Geometry check sheet. Reference: the model listing, model coordinates, mm. A direction names the side the tool comes from. Round coordinates to 2 decimals unless told otherwise and drop trailing zeros. Order: outer loops, then holes, each group sorted by start corner. A loop starts at its lowest first (then second) coordinate and runs counter-clockwise, first axis right, second up.
```python
from build123d import *

# Parameters (mm, degrees)
SKETCH1_W           = 66
SKETCH1_H           = 49
BOSS_EXTRUDE1_DEPTH = 19
SHELL1_T            = -1.5
SKETCH2_W           = 6
SKETCH2_H           = 4.6
BOSS_EXTRUDE2_DEPTH = 17.5
FILLET1_R           = 1.5
SKETCH3_R           = 2.15
SKETCH3_R_2         = 1.45
BOSS_EXTRUDE3_DEPTH = 4.6
BOSS_EXTRUDE4_DEPTH = 0.5
FILLET2_R           = 4
FILLET3_R           = 2
BOSS_EXTRUDE5_REACH = 351.368
SKETCH5_R           = 3.5
FILLET4_R           = 2


with BuildPart() as part:
    # Sketch1 → Boss-Extrude1 (new body)
    with BuildSketch(Plane.XY.offset(30)):
        with Locations((105.809562907, 295.544660887)):
            Rectangle(SKETCH1_W, SKETCH1_H)
    extrude(amount=BOSS_EXTRUDE1_DEPTH)

    # Shell1
    shell1_openings = [part.faces().sort_by_distance(p)[0] for p in [
        (105.809562907, 295.544660887, 49),
    ]]
    offset(amount=SHELL1_T, openings=shell1_openings, kind=Kind.INTERSECTION)

    # Sketch2 → Boss-Extrude2 (add)
    with BuildSketch(Plane.XY.offset(31.5)):
        with Locations((90.011318394, 316.244660887)):
            Rectangle(SKETCH2_W, SKETCH2_H)
        with Locations((121.756668801, 316.244660887)):
            Rectangle(SKETCH2_W, SKETCH2_H)
    extrude(amount=BOSS_EXTRUDE2_DEPTH)

    # Fillet1
    fillet1_edges = [part.edges().sort_by_distance(p)[0] for p in [
        (74.309562907, 318.544660887, 40.25),
        (137.309562907, 318.544660887, 40.25),
        (72.809562907, 320.044660887, 39.5),
        (138.809562907, 320.044660887, 39.5),
    ]]
    fillet(fillet1_edges, radius=FILLET1_R)

    # Sketch3 → Boss-Extrude3 (add)
    # profile 1 of 4: a face of its own
    with BuildSketch(Plane.XY.offset(31.5)):
        with Locations((90.939840403, 307.111410879)):
            Circle(SKETCH3_R)
        with Locations((90.939840403, 307.111410879)):
            Circle(SKETCH3_R_2, mode=Mode.SUBTRACT)
    # profile 2 of 4: a face of its own
    with BuildSketch(Plane.XY.offset(31.5)):
        with Locations((120.939840403, 307.111410879)):
            Circle(SKETCH3_R)
        with Locations((120.939840403, 307.111410879)):
            Circle(SKETCH3_R_2, mode=Mode.SUBTRACT)
    # profile 3 of 4: a face of its own
    with BuildSketch(Plane.XY.offset(31.5)):
        with Locations((120.939840403, 292.111410879)):
            Circle(SKETCH3_R)
        with Locations((120.939840403, 292.111410879)):
            Circle(SKETCH3_R_2, mode=Mode.SUBTRACT)
    # profile 4 of 4: a face of its own
    with BuildSketch(Plane.XY.offset(31.5)):
        with Locations((90.939840403, 292.111410879)):
            Circle(SKETCH3_R)
        with Locations((90.939840403, 292.111410879)):
            Circle(SKETCH3_R_2, mode=Mode.SUBTRACT)
    extrude(amount=BOSS_EXTRUDE3_DEPTH)

    # Sketch4 → Boss-Extrude4 (add, symmetric)
    with BuildSketch(Plane(origin=(0, 284, 0), x_dir=(1, 0, 0), z_dir=(0, 1, 0))):
        Polygon((72.809562907, -47.615589413), (78.809562907, -47.615589413), (78.809562907, -37.615589413), (132.809562907, -37.615589413), (132.809562907, -47.615589413), (138.809562907, -47.615589413), (138.809562907, -30), (72.809562907, -30), align=None)
    extrude(amount=BOSS_EXTRUDE4_DEPTH, both=True)

    # Fillet2
    fillet2_edges = [part.edges().sort_by_distance(p)[0] for p in [
        (78.809562907, 284, 47.615589413),
        (132.809562907, 284, 47.615589413),
    ]]
    fillet(fillet2_edges, radius=FILLET2_R)

    # Fillet3
    fillet3_edges = [part.edges().sort_by_distance(p)[0] for p in [
        (78.809562907, 284, 37.615589413),
        (132.809562907, 284, 37.615589413),
    ]]
    fillet(fillet3_edges, radius=FILLET3_R)

    # Boss-Extrude5: up to this face of the body (flat: up to its plane)
    boss_extrude5_end = Plane(part.part.faces().sort_by_distance((105.809562907, 295.537442811, 30))[0])
    # Sketch5 → Boss-Extrude5 (add, up to the picked face)
    with BuildSketch(Plane.XY.offset(49), mode=Mode.PRIVATE) as boss_extrude5_sk1:
        with Locations((76.56102911, 270.299359986)):
            Circle(SKETCH5_R)
    boss_extrude5_tool1 = split(extrude(boss_extrude5_sk1.sketch, amount=-BOSS_EXTRUDE5_REACH, mode=Mode.PRIVATE), bisect_by=boss_extrude5_end, keep=Keep.BOTH, mode=Mode.PRIVATE)
    # Sketch5 → Boss-Extrude5 (add, up to the picked face)
    with BuildSketch(Plane.XY.offset(49), mode=Mode.PRIVATE) as boss_extrude5_sk2:
        with Locations((135, 270)):
            Circle(SKETCH5_R)
    boss_extrude5_tool2 = split(extrude(boss_extrude5_sk2.sketch, amount=-BOSS_EXTRUDE5_REACH, mode=Mode.PRIVATE), bisect_by=boss_extrude5_end, keep=Keep.BOTH, mode=Mode.PRIVATE)
    add(boss_extrude5_tool1.solids().sort_by(Axis((76.561029, 270.29936, 49), (0, 0, -1)))[0])
    add(boss_extrude5_tool2.solids().sort_by(Axis((135, 270, 49), (0, 0, -1)))[0])

    # Fillet4
    fillet4_edges = [part.edges().sort_by_distance(p)[0] for p in [
        (79.980755206, 271.044660887, 39.5),
        (131.659538411, 271.044660887, 39.5),
        (87.011318394, 313.944660887, 40.25),
        (93.011318394, 313.944660887, 40.25),
        (118.756668801, 313.944660887, 40.25),
        (124.756668801, 313.944660887, 40.25),
    ]]
    fillet(fillet4_edges, radius=FILLET4_R)


solid = part.part
```
(1) Depth check by flat-ended pin: P1, Ø3.5, axis at x = 120.94, y = 292.11, coming from the +Z side; P2, Ø5, axis at x = 131.5, z = 39.5, coming from the -Y side; P3, Ø9, axis at x = 82.5, z = 36.5, coming from the -Y side. Enter the tip coordinate at first touch or a pass-through.
Returned:
P1: stops at z = 36.1
P2: stops at y = 266.65
P3: stops at y = 267.11
(2) Sectioned sample at A-A, the plane x = 103. Record the cut outline in (y, z), and give its area (3 significant figures).
Returned:
outline: (271.04, 30) - (320.04, 30) - (320.04, 49) - (318.54, 49) - (318.54, 31.5) - (284.5, 31.5) - (284.5, 37.62) - (283.5, 37.62) - (283.5, 31.5) - (272.54, 31.5) - (272.54, 49) - (271.04, 49) - close
area: 132 mm2
(3) Set-up check for faces 5 (the cylindrical face through (73.237, 319.594, 39.633)), 6 (the flat face through (106, 272.545, 40)): record each of +Z, -Z, +X, -X, +Y, -Y from which the full face is reachable in a straight line by a thin tool's end or side.
Returned:
face 5: +Z, -Z, -X, +Y
face 6: +Z
(4) Material ranges on line 1 (Y direction, x = 100, z = 35.5); line 2 (X direction, y = 287.5, z = 45.5); line 3 (Y direction, x = 90, z = 44.25), recorded low to high.
Returned:
line 1: y = 271.04 to 272.54, 283.5 to 284.5, 318.54 to 320.04
line 2: x = 72.81 to 74.31, 137.31 to 138.81
line 3: y = 271.04 to 272.54, 313.94 to 320.04
(5) Draft check along Y on faces 1 (the cylindrical face through (91.609, 305.825, 33.768)), 2 (the flat face through (106, 294, 30)), 3 (the cylindrical face through (130.884, 270.564, 39.633)), 4 (the flat face through (105, 320.045, 39)). Enter one of: released by +Y, released by -Y, zero draft, split by the parting line, or undercut.
Returned:
face 1: undercut
face 2: zero draft
face 3: released by -Y
face 4: released by +Y
(6) Sectioned sample at C-C, the plane x = 135. Record the cut outline in (y, z).
Returned:
outline: (266.5, 30) - (320.04, 30) - (320.04, 49) - (318.54, 49) - (318.54, 31.5) - (284.5, 31.5) - (284.5, 47.18) - (283.5, 47.18) - (283.5, 31.5) - (273.5, 31.5) - (273.5, 49) - (266.5, 49) - close
(7) Sectioned sample at B-B, the plane y = 299.5. Record the cut outline in (x, z).
Returned:
outline: (72.81, 30) - (138.81, 30) - (138.81, 49) - (137.31, 49) - (137.31, 31.5) - (74.31, 31.5) - (74.31, 49) - (72.81, 49) - close
